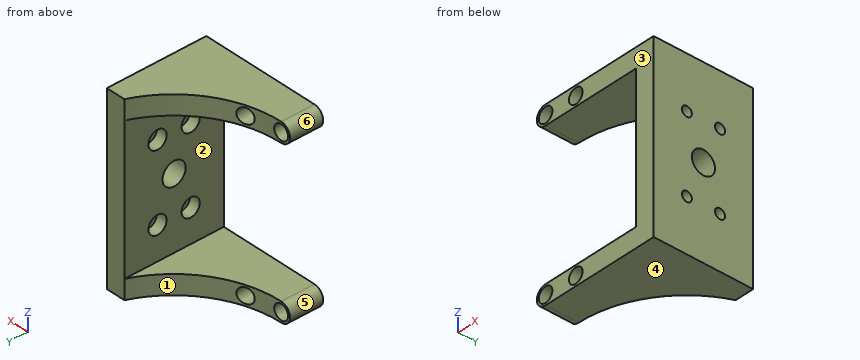
Autodesk Inventor part; units mm, degrees
ref_plane "Work Plane1" through (25, 10, 10.0475) normal (0, 0, -1) x (-1, 0, 0)
ref_plane "YZ Plane" through (0, 0, 0) normal (1, 0, 0) x (0, 1, 0)
ref_plane "XZ Plane" through (0, 0, 0) normal (0, 1, 0) x (-1, 0, 0)
sketch "Sketch1" plane through (0, 0, 0) normal (0, 1, 0) x (-1, 0, 0)
  circle A0 centre (-5, -14.4525) radius 2.25
  circle A1 centre (5, -14.4525) radius 2.25
  circle A2 centre (5, 34.5475) radius 2.25
  circle A3 centre (-5, 34.5475) radius 2.25
  line L0 (21.75, 43.0475) -> (-21.75, 43.0475)
  line L1 (21.75, -42.9525) -> (21.75, 43.0475)
  line L2 (-21.75, 43.0475) -> (-21.75, -42.9525)
  line L3 (-21.75, 43.0475) -> (21.75, 43.0475)
  line L4 (21.75, 43.0475) -> (21.75, -42.9525)
  line L5 (21.75, -42.9525) -> (-21.75, -42.9525)
  line L6 (-21.75, -42.9525) -> (-21.75, 43.0475)
  circle A4 centre (-5, 34.5475) radius 2.9
  circle A5 centre (5, 34.5475) radius 2.9
  circle A6 centre (-5, -14.4525) radius 2.9
  circle A7 centre (5, -14.4525) radius 2.9
  line L7 (5, 37.4475) -> (-5, 37.4475)
  line L8 (5, 31.6475) -> (-5, 31.6475)
  line L9 (5, -11.5525) -> (-5, -11.5525)
  line L10 (5, -17.3525) -> (-5, -17.3525)
  line L11 (-5, 37.4475) -> (-30.8, 37.4475)
  line L12 (-5, -17.3525) -> (-30.8, -17.3525)
  line L13 (-30.8, -17.3525) -> (-30.8, 37.4475)
  line L14 (-5, 31.6475) -> (-25, 31.6475)
  line L15 (-25, 31.6475) -> (-25, -11.5525)
  line L16 (-25, -11.5525) -> (-5, -11.5525)
  point P0 (0, 0)
  point P1 (-1.4735, -1.6316)
  dimension "d0" = 5.8
  dimension "d1" = 5.8
  dimension "d2" = 5.8
  dimension "d3" = 5.8
  dimension "d4" = 4.5
  dimension "d5" = 4.5
  dimension "d6" = 4.5
  dimension "d7" = 4.5
  dimension "d8" = 25.8
  dimension "d9" = 20
extrude "Extrusion1" add sketch "Sketch1" along normal blind 10 contours L11 A4 L14 L2 | L2 L14 L15 L16 L12 L13 L11 | L7 A5 L8 A4 | A4 | L2 L16 A6 L12 | A5 | A6 | A6 L9 A7 L10 | A7
sketch "Sketch2" plane through (25, 0, -11.5525) normal (-1, 0, 0) x (0, 0, 1)
  line L0 (0, 0) -> (0, 10)
  line L1 (43.2, 0) -> (43.2, 10)
  line L2 (0, 10) -> (43.2, 10)
  line L3 (43.2, 10) -> (43.2, 30)
  line L4 (43.2, 30) -> (0, 30)
  line L5 (0, 30) -> (0, 10)
  point P0 (11.5525, 0)
  dimension "d12" = 20
extrude "Extrusion2" add sketch "Sketch2" against normal up to surface (5.8 mm away)
sketch "Sketch3" plane through (25, 0, -11.5525) normal (-1, 0, 0) x (0, 0, 1)
  line L0 (0, 0) -> (43.2, 0)
  line L1 (43.2, 0) -> (43.2, 10)
  line L2 (43.2, 10) -> (43.2, 30)
  line L3 (43.2, 30) -> (0, 30)
  line L4 (0, 30) -> (0, 10)
  line L5 (0, 0) -> (0, 10)
  circle A0 centre (10, 10) radius 2.75
  line L6 (0, 30) -> (43.2, 30)
  line L7 (43.2, 30) -> (43.2, 0)
  line L8 (43.2, 0) -> (0, 0)
  line L9 (0, 0) -> (0, 30)
  circle A1 centre (10, 20) radius 2.75
  circle A2 centre (33.2, 20) radius 2.75
  circle A3 centre (33.2, 10) radius 2.75
  point P0 (11.5525, 0)
  dimension "d15" = 5.5
  dimension "d16" = 10
  dimension "d17" = 10
  dimension "d18" = 5.5
  dimension "d19" = 5.5
  dimension "d20" = 10
  dimension "d21" = 5.5
  dimension "d22" = 43.2
  dimension "d23" = 30
extrude "Extrusion3" cut sketch "Sketch3" against normal blind 3.2 contours A0 | A1 | A2 | A3
sketch "Sketch4" plane through (25, 0, -11.5525) normal (-1, 0, 0) x (0, 0, 1)
  circle A0 centre (10, 10) radius 2.75
  circle A1 centre (10, 10) radius 1.5
  circle A2 centre (10, 20) radius 2.75
  circle A3 centre (10, 20) radius 1.5
  circle A4 centre (33.2, 10) radius 2.75
  circle A5 centre (33.2, 20) radius 2.75
  circle A6 centre (33.2, 10) radius 1.5
  circle A7 centre (33.2, 20) radius 1.5
  point P0 (11.5525, 0)
  dimension "d26" = 3
  dimension "d27" = 3
  dimension "d28" = 3
  dimension "d29" = 3
extrude "Extrusion4" cut sketch "Sketch4" against normal blind 10 contours A1 | A3 | A6 | A7
sketch "Sketch5" plane through (25, 10, 31.6475) normal (0, 0, 1) x (1, 0, 0)
  line L0 (3.2, 7.25) -> (3.2, 12.75)
  line L1 (5.8, 0) -> (5.8, 20)
  line L2 (0, 20) -> (5.8, 20)
  line L3 (0, 0) -> (0, 20)
  line L4 (5.8, 0) -> (0, 0)
  line L5 (-30, -10) -> (5.8, -10)
  line L6 (5.8, -10) -> (5.8, 0)
  line L7 (-30, 0) -> (5.8, 0)
  line L8 (-30, -10) -> (-30, 0)
  line L9 (-30, -10) -> (-30, 0)
  arc A0 (-30, 0) -> (0, 20) centre (-30, 32.5) ccw
  line L10 (-30, 0) -> (5.8, 0)
  line L11 (-30, 0) -> (0, 0)
  line L12 (-32.9, -10) -> (-32.9, 0)
  line L13 (0, 20) -> (0, 0)
  point P0 (-25, -10)
extrude "Extrusion5" add sketch "Sketch5" along normal up to surface (5.8 mm away) contours L4 L3 L2 L1 | L7 A0 L3
ref_plane "Work Plane1" through (25, 10, 10.0475) normal (0, 0, -1) x (-1, 0, 0)
mirror "Mirror1" about plane through (25, 10, 10.0475) normal (0, 0, -1) of "Extrusion5"
extrude "Extrusion6" cut sketch "Sketch1" along normal blind 33.8125 contours A0 | A1 | A2 | A3
sketch "Sketch6" plane through (25, 0, -11.5525) normal (-1, 0, 0) x (0, 0, 1)
  circle A0 centre (33.2, 10) radius 2.75
  circle A1 centre (10, 10) radius 2.75
  circle A2 centre (33.2, 20) radius 2.75
  circle A3 centre (10, 20) radius 2.75
  line L0 (0, 0) -> (43.2, 0)
  line L1 (43.2, 0) -> (43.2, 30)
  line L2 (43.2, 30) -> (0, 30)
  line L3 (0, 0) -> (0, 30)
  line L4 (10, 20) -> (33.2, 10) construction
  line L5 (33.2, 20) -> (10, 10) construction
  circle A4 centre (21.6, 15) radius 3.5
  point P0 (11.5525, 0)
  dimension "d37" = 7
extrude "Extrusion7" cut sketch "Sketch6" against normal through all contours A4
properties part number "SERVO_TO_TOOLHEAD_3DPrint"
Source: CAD feature listing. Evaluate the final solid. Frame: model axes, mm. Face numbers are marked on the shaded views. A direction names the side the tool comes from. Coordinates: 2 decimals unless noted, no trailing zeros. Loops run counter-clockwise (first coordinate to the right, second up) from the corner with the lowest first, then second, coordinate; pieces in that order, holes last. Notation, with made-up numbers: (-13.5, -20) - (3.5, -20) arc R11 ccw to (3.5, 0) - close; hole circle Ø2 at (-0.5, 56.5). An arc over 180 degrees is marked (long way). One line per item, written item: value. Start each with the question number.
1. Section C-C (x = -2). Return the cut outline in (y, z).
2. Ray query, L1, parallel to Z at x = 5, y = 3.5; L2, parallel to Z at x = 11.5, y = 4; L3, parallel to X at y = 3, z = 34. Return the intervals inside material, ascending.
3. Section A-A (x = 26.5). Return the cut outline in (y, z).
4. Mould query, pull axis Z, two halves, no side actions, for the marked faces 3, 4, 5 and 6. Classes: pulls with the +Z half, pulls with the -Z half, needs draft (parallel to the pull), parting line crosses it, or undercut.
5. Section D-D (y = 15). Return the cut outline in (x, z), and give its area (3 significant figures).
6. Set-up query: the marked faces 1 and 2. Return all of +Z, -Z, +X, -X, +Y, -Y with unobstructed straight access to the full face (end or side cutting, diameter ignored); none if empty.
7. Contact query for flat-ended pins moving along their axis: P1, Ø3.5, axis at x = 5, z = 34.55, coming from the +Y side; P2, Ø6, axis at y = 21, z = 20.5, coming from the -X side; P3, Ø3.5, axis at y = 20, z = 21.65, coming from the -X side; P4, Ø2.5, axis at x = -6.5, z = 35, coming from the +Y side. Output: stop coordinate, or through.
8. Section B-B (y = 20). Return the cut outline in (x, z), and give its area (3 significant figures).
Verdict:
1. outline: (0, -17.35) - (10.14, -17.35) - (10.14, -11.55) - (0, -11.55) - close; (0, 31.65) - (10.14, 31.65) - (10.14, 37.45) - (0, 37.45) - close
2. L1: z = -17.35 to -16.7, -12.2 to -11.55, 31.65 to 32.3, 36.8 to 37.45
2. L2: z = -17.35 to -11.55, 31.65 to 37.45
2. L3: x = -7.85 to -7.18, -2.82 to 2.82, 7.18 to 30.8
3. outline: (0, -17.35) - (30, -17.35) - (30, 37.45) - (0, 37.45) - close; hole circle Ø5.5 at (10, -1.55); hole circle Ø5.5 at (10, 21.65); hole circle Ø7 at (15, 10.05); hole circle Ø5.5 at (20, -1.55); hole circle Ø5.5 at (20, 21.65)
4. face 3: needs draft
4. face 4: pulls with the -Z half
4. face 5: undercut
4. face 6: undercut
5. outline: (12.32, -17.35) - (30.8, -17.35) - (30.8, 6.55) - (25, 6.55) - (25, -11.55) - (12.32, -11.55) - close; (12.32, 31.65) - (25, 31.65) - (25, 13.55) - (30.8, 13.55) - (30.8, 37.45) - (12.32, 37.45) - close
5. area: 424 mm2
6. face 1: +Z, -Z, -X, +Y
6. face 2: -X, +Y, -Y
7. P1: passes through
7. P2: stops at x = 25
7. P3: stops at x = 28.2
7. P4: stops at y = 10
8. outline: (18.45, -17.35) - (30.8, -17.35) - (30.8, -3.05) - (28.2, -3.05) - (28.2, -4.3) - (25, -4.3) - (25, -11.55) - (18.45, -11.55) - close; (18.45, 31.65) - (25, 31.65) - (25, 24.4) - (28.2, 24.4) - (28.2, 23.15) - (30.8, 23.15) - (30.8, 37.45) - (18.45, 37.45) - close; (25, 1.2) - (28.2, 1.2) - (28.2, -0.05) - (30.8, -0.05) - (30.8, 20.15) - (28.2, 20.15) - (28.2, 18.9) - (25, 18.9) - close
8. area: 343 mm2
